Source: CAD feature listing. Evaluate the final solid. Frame: model axes, mm. A direction names the side the tool comes from. Give positions to 0.01 mm unless a question says otherwise; leave off trailing zeros. Order: outer loops, then holes, each group sorted by start corner. A loop starts at its lowest first (then second) coordinate and runs counter-clockwise, first axis right, second up. Notation, with made-up numbers: (51, 54) -> (85, 54) arc R12 ccw to (85, 68) -> close; hole circle Ø5 at (30.5, 36). An arc over 180 degrees is marked (long way). Answer in a Markdown table with one row per item.
Autodesk Inventor part; units mm, degrees
ref_plane "Work Plane1" through (-19.5008, 0, -114.8484) normal (0, 0, -1) x (-1, 0, 0)
ref_plane "Work Plane2" through (-19.5008, 0, -89.8484) normal (0, 0, -1) x (-1, 0, 0)
ref_plane "Work Plane3" through (-24.9546, 0, -79.8533) normal (0, 0, -1) x (-1, 0, 0)
sketch "Sketch1" plane through (0, 0, 0) normal (0, 1, 0) x (-1, 0, 0)
  line L0 (-0.0661, 0.1517) -> (59.9339, 0.1517)
  line L1 (59.9339, 0.1517) -> (59.9339, -119.8483)
  line L2 (59.9339, -119.8483) -> (-0.0661, -119.8483)
  line L3 (-0.0661, -119.8483) -> (-0.0661, 0.1517)
  line L4 (29.9339, -119.8483) -> (29.9339, 0.1517)
  circle A0 centre (29.9339, -54.8547) radius 22.5
  line L5 (19.5008, -89.8484) -> (19.5008, -114.8484)
  line L6 (19.5008, -114.8484) -> (40.5008, -114.8484)
  line L7 (40.5008, -114.8484) -> (40.5008, -89.8484)
  line L8 (40.5008, -89.8484) -> (19.5008, -89.8484)
  line L9 (19.5008, -89.8484) -> (40.5008, -114.8484) construction
  line L10 (19.5008, -114.8484) -> (40.5008, -89.8484) construction
  line L11 (19.5008, -89.8484) -> (44.5008, -89.8484) construction
  line L12 (24.9546, -79.8533) -> (24.9546, -89.8533)
  line L13 (24.9546, -89.8533) -> (34.9546, -89.8533)
  line L14 (34.9546, -89.8533) -> (34.9546, -79.8533)
  line L15 (34.9546, -79.8533) -> (24.9546, -79.8533)
  line L16 (24.9546, -79.8533) -> (34.9546, -89.8533) construction
  line L17 (24.9546, -89.8533) -> (34.9546, -79.8533) construction
  line L18 (24.9546, -79.8533) -> (34.9546, -79.8533) construction
  line L19 (7.4339, -10.8533) -> (7.4339, -79.8533)
  line L20 (7.4339, -79.8533) -> (52.4339, -79.8533)
  line L21 (52.4339, -79.8533) -> (52.4339, -10.8533)
  line L22 (52.4339, -10.8533) -> (7.4339, -10.8533)
  line L23 (7.4339, -10.8533) -> (52.4339, -79.8533) construction
  line L24 (7.4339, -79.8533) -> (52.4339, -10.8533) construction
  line L25 (7.4339, -10.8533) -> (76.4339, -10.8533) construction
  line L26 (34.9339, -5.8533) -> (24.9339, -5.8533)
  line L27 (24.9339, -5.8533) -> (24.9339, -15.8533)
  line L28 (24.9339, -15.8533) -> (34.9339, -15.8533)
  line L29 (34.9339, -15.8533) -> (34.9339, -5.8533)
  line L30 (34.9339, -5.8533) -> (24.9339, -15.8533) construction
  line L31 (24.9339, -5.8533) -> (34.9339, -15.8533) construction
  point P0 (0, 0)
  point P1 (29.9339, -114.8483)
  point P2 (30.4342, -89.8533)
  point P3 (29.9546, -89.8533)
  point P4 (29.9339, -79.8533)
  point P5 (30.0136, -77.3546)
  point P6 (29.9339, -25)
  point P7 (30.0008, -102.3484)
  point P8 (29.9339, -10.8533)
  point P9 (29.9546, -84.8533)
  point P10 (29.9339, -10.8533)
  point P11 (29.9339, -45.3533)
  point P12 (34.9546, -79.8533)
  point P13 (24.9546, -79.8533)
  point P14 (24.9546, -89.8484)
  point P15 (34.9546, -89.8484)
  point P16 (34.9339, -10.8533)
  point P17 (24.9339, -10.8533)
  dimension "d0" = 60
  dimension "d1" = 120
  dimension "d2" = 45
  dimension "d3" = 5
  dimension "d4" = 25
  dimension "d6" = 12.5
  dimension "d7" = 10
  dimension "d8" = 2.5
  dimension "d9" = 22.5
  dimension "d10" = -69
  dimension "d11" = 25
  dimension "d12" = 90
  dimension "d13" = 21
  dimension "d14" = 5
  dimension "d15" = 10
  dimension "d16" = 90
  dimension "d17" = 10
  dimension "d18" = -69
  dimension "d19" = 90
  dimension "d20" = -34.5
  dimension "d21" = 45
  dimension "d42" = 10
  dimension "d43" = 10
extrude "Extrusion1" add sketch "Sketch1" against normal blind 60
sketch "Sketch2" plane through (0.0661, 0, -119.8483) normal (0, 0, -1) x (-1, 0, 0)
  line L0 (0, 0) -> (60, 0)
  line L1 (0, 0) -> (0, -60)
  line L2 (60, -60) -> (0, -60)
  line L3 (60, 0) -> (60, -60)
  point P0 (0.0661, 0)
  point P1 (30, -30)
ref_plane "Work Plane1" through (-19.5008, 0, -114.8484) normal (0, 0, -1) x (-1, 0, 0)
ref_plane "Work Plane2" through (-19.5008, 0, -89.8484) normal (0, 0, -1) x (-1, 0, 0)
ref_plane "Work Plane3" through (-24.9546, 0, -79.8533) normal (0, 0, -1) x (-1, 0, 0)
ref_plane "Work Plane5" through (-7.4339, 0, -5.8533) normal (0, 0, -1) x (-1, 0, 0)
ref_plane "Work Plane4" through (-7.4339, 0, -10.8533) normal (0, 0, -1) x (-1, 0, 0)
sketch "Sketch3" plane through (-19.5008, 0, -114.8484) normal (0, 0, -1) x (-1, 0, 0)
  circle A0 centre (10.433, -30) radius 10.5
  point P0 (-19.5008, 0)
  dimension "d25" = 21
ref_plane "Work Plane6" through (-29.9339, -30, -119.8483) normal (0, 1, 0) x (1, 0, 0)
extrude "Extrusion3" cut sketch "Sketch1" against normal up to surface (30 mm away) contours L22 L29 L28 L4 | L4 L28 L27 L22 | L6 L5 L8 L12 L13 L4 | L4 L13 L14 L8 L7 L6 | L28 L29 L22 L21 A0 L4 | L4 A0 L19 L22 L27 L28 | L13 L12 L8 L4 | L4 L8 L14 L13 | A0 L4 | L4 A0 | L8 L12 L15 L4 | L4 L15 L14 L8 | A0 L21 L20 L15 L4 | L4 L15 L20 L19 A0
sketch "Sketch4" plane through (-19.5008, 0, -89.8484) normal (0, 0, -1) x (-1, 0, 0)
  circle A0 centre (10.433, -30) radius 5
  point P0 (-19.5008, 0)
  point P1 (15.4537, 0)
  point P2 (15.4537, 0)
  point P3 (15.4537, 0)
  point P4 (5.4537, 0)
  point P5 (5.4537, 0)
  point P6 (5.4537, 0)
  dimension "d30" = 10
sketch "Sketch5" plane through (-24.9546, 0, -79.8533) normal (0, 0, -1) x (-1, 0, 0)
  circle A0 centre (4.9793, -30) radius 22.5
  point P0 (-24.9546, 0)
  dimension "d31" = 45
extrude "Extrusion4" cut sketch "Sketch3" against normal up to surface (25 mm away)
ref_plane "Work Plane7" through (0.0661, 0, -117.8483) normal (0, 0, -1) x (-1, 0, 0)
extrude "Extrusion5" cut sketch "Sketch4" against normal up to surface (83.9952 mm away)
extrude "Extrusion6" cut sketch "Sketch5" against normal up to surface (69 mm away)
extrude "Extrusion7" cut sketch "Sketch4" along normal up to surface (27.9998 mm away)
fillet "Fillet1" radius 2 4 edges at (-59.9339, -30, 0.1517) (0.0661, -30, 0.1517) (0.0661, -30, -119.8483) (-59.9339, -30, -119.8483)
extrude "Extrusion8" cut sketch "Sketch1" against normal through all contours L22 L29 L28 L4 | L4 L28 L27 L22
chamfer "Chamfer1" distance 2 angle 45 4 edges at (-29.9339, -60, -10.8533) (-24.9339, -60, -13.3533) (-29.9339, -60, -15.8533) (-34.9339, -60, -13.3533)
chamfer "Chamfer2" distance 2 angle 45 3 edges at (-34.9339, -51.9374, -13.3533) (-29.9339, -52.5, -15.8533) (-24.9339, -51.9374, -13.3533)
fillet "Fillet2" radius 1 1 edges at (-24.9339, -30, -114.8484)
fillet "Fillet3" radius 1 1 edges at (-24.9339, -30, -10.8533)
sketch "Sketch6" plane through (0, -60, 0) normal (0, -1, 0) x (1, 0, 0)
  arc A0 (-59.9339, -117.8483) -> (-57.9339, -119.8483) centre (-57.9339, -117.8483) ccw
  line L0 (-57.9339, -119.8483) -> (-1.9339, -119.8483)
  arc A1 (-1.9339, -119.8483) -> (0.0661, -117.8483) centre (-1.9339, -117.8483) ccw
  line L1 (0.0661, -117.8483) -> (0.0661, -1.8483)
  arc A2 (0.0661, -1.8483) -> (-1.9339, 0.1517) centre (-1.9339, -1.8483) ccw
  line L2 (-1.9339, 0.1517) -> (-57.9339, 0.1517)
  arc A3 (-57.9339, 0.1517) -> (-59.9339, -1.8483) centre (-57.9339, -1.8483) ccw
  line L3 (-59.9339, -1.8483) -> (-59.9339, -117.8483)
  line L4 (-36.9339, -8.8533) -> (-36.9339, -17.8533)
  line L5 (-22.9339, -8.8533) -> (-36.9339, -8.8533)
  line L6 (-22.9339, -17.8533) -> (-22.9339, -8.8533)
  line L7 (-36.9339, -17.8533) -> (-22.9339, -17.8533)
  line L8 (-29.9339, 0.1517) -> (-29.9339, -119.8483)
  line L9 (0.0661, -59.8483) -> (-59.9339, -59.8483)
  line L10 (-29.9339, -59.8483) -> (-29.9339, -119.8483)
  line L11 (-29.9339, -59.8483) -> (-29.9339, -89.8483)
  line L12 (-29.9339, -89.8483) -> (-29.9339, -119.8483)
  line L13 (-29.9339, -89.8483) -> (-59.9339, -89.8483)
  line L14 (-59.9339, -89.8483) -> (-59.9339, -119.8483)
  line L15 (-59.9339, -119.8483) -> (-29.9339, -119.8483)
  line L16 (-29.9339, -119.8483) -> (-29.9339, -89.8483)
  circle A4 centre (-44.9339, -104.8483) radius 3.75
  circle A5 centre (-14.9339, -104.8483) radius 3.75
  circle A6 centre (-44.9339, -74.8483) radius 3.75
  circle A7 centre (-14.9339, -74.8483) radius 3.75
  point P0 (0, 0)
  point P1 (-29.9339, -74.8483)
  point P2 (-29.9339, -104.8483)
  dimension "d58" = 7.5
  dimension "d61" = 30
  dimension "d64" = 30
extrude "Extrusion10" add sketch "Sketch6" along normal blind 5 contours A4 | A5 | A6 | A7
equation "\"d18\" = d10"
equation "\"d21\" = d2"
equation "\"d31\" = d2"
properties part number "housing_V2_3DPrint"
(1) Section query D-D (z = -72.5). Return the cut outline in (x, y), plus the area to 3 significant figures.
A:
| item | result |
|---|---|
| outline | (-59.93, -60) -> (-47.86, -60) -> (-47.86, -65) -> (-42.01, -65) -> (-42.01, -60) -> (-17.86, -60) -> (-17.86, -65) -> (-12.01, -65) -> (-12.01, -60) -> (0.07, -60) -> (0.07, 0) -> (-7.43, 0) -> (-7.43, -30) arc R22.5 cw to (-52.43, -30) -> (-52.43, 0) -> (-59.93, 0) -> close |
| area | 1,510 mm^2 |
(2) Access query for faces 4 (the flat face through (-24.934, -56, -13)), 5 (the flat face through (-19.501, -14, -102)), 6 (the flat face through (-30, -30, -5.853)), 7 (the cylindrical face through (-11.47, -62.46, -103.41)). Directions: +Z, -Z, +X, -X, +Y, -Y. A direction counts if a zero-diameter tool reaches every point of the face in a straight line with its end or side. Return the directions, or none.
A:
| item | result |
|---|---|
| face 4 | +Y, -Y |
| face 5 | +Y |
| face 6 | none |
| face 7 | -Y |
(3) Ray query, probe 1 along Z at (x, y) = (-37, -5); probe 2 along X at (y, z) = (-30, -7.95); probe 3 along X at (y, z) = (-26, -87). Return the intervals inside material, ascending.
A:
| item | result |
|---|---|
| probe 1 | z = -119.85 to -114.85, -89.85 to -79.85, -10.85 to 0.15 |
| probe 2 | x = -59.93 to -34.93, -24.93 to 0.07 |
| probe 3 | x = -59.93 to -34.95, -24.95 to 0.07 |
(4) Section query A-A (z = -26). Return the cut outline in (x, y), plus the area to 3 significant figures.
A:
| item | result |
|---|---|
| outline | (-59.93, -60) -> (0.07, -60) -> (0.07, 0) -> (-7.43, 0) -> (-7.43, -30) arc R22.5 cw to (-52.43, -30) -> (-52.43, 0) -> (-59.93, 0) -> close |
| area | 1,450 mm^2 |
(5) Section query C-C (x = -55). Return the cut outline in (y, z), plus the area to 3 significant figures.
A:
| item | result |
|---|---|
| outline | (-60, -119.85) -> (0, -119.85) -> (0, 0.15) -> (-60, 0.15) -> close |
| area | 7,200 mm^2 |
(6) Section query B-B (x = -43). Return the cut outline in (y, z).
A:
| item | result |
|---|---|
| outline | (-65, -108.06) -> (-60, -108.06) -> (-60, -119.85) -> (0, -119.85) -> (0, -79.85) -> (-48.32, -79.85) -> (-48.32, -10.85) -> (0, -10.85) -> (0, 0.15) -> (-60, 0.15) -> (-60, -71.64) -> (-65, -71.64) -> (-65, -78.06) -> (-60, -78.06) -> (-60, -101.64) -> (-65, -101.64) -> close |
(7) First-contact query: pin 1 Ø4 at (x, z) = (-15, -73) entering from +Y. Flat tip, straight axial feed; report the tip coordinate or a pass-through.
A:
| item | result |
|---|---|
| pin 1 | stops at y = -44.82 |
(8) Pull-direction query (X, two-part tool) for faces 1 (the flat face through (-30, -56, -15.853)), 2 (the flat face through (-59.934, -30, -59)), 3 (the flat face through (-45, -65, -75)); classes: +X half, -X half, draft (parallel to the pull), parting line (faces both ways), or undercut.
A:
| item | result |
|---|---|
| face 1 | undercut |
| face 2 | -X half |
| face 3 | draft |
